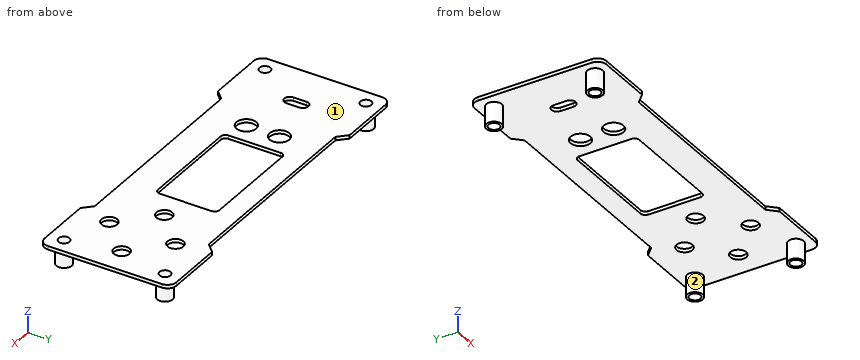
from build123d import *

# Parameters (mm, degrees)
PAD_DEPTH       = 0.8
POCKET_DEPTH    = 0.801
POCKET001_DEPTH = 0.801
SKETCH002_R     = 2.25
POCKET002_DEPTH = 0.801
SKETCH003_R     = 1.8
POCKET003_DEPTH = 0.801
SKETCH004_R     = 1.75
PAD001_DEPTH    = 4.5
SKETCH005_R     = 1.25
POCKET004_DEPTH = 5.301


with BuildPart() as part:
    # PCB_Sketch_76c7 → Pad (new body)
    with BuildSketch(Plane.XY):
        with BuildLine():
            Line((80, 28), (80, 2))
            ThreePointArc((80, 2), (79.414214, 0.585786), (78, 0))
            Line((78, 0), (65, 0))
            Line((65, 0), (63, 2))
            Line((63, 2), (17, 2))
            Line((17, 2), (15, 0))
            Line((15, 0), (2, 0))
            ThreePointArc((2, 0), (0.585786, 0.585786), (0, 2))
            Line((0, 2), (0, 28))
            ThreePointArc((0, 28), (0.585786, 29.414214), (2, 30))
            Line((2, 30), (15, 30))
            Line((17, 28), (15, 30))
            Line((63, 28), (17, 28))
            Line((63, 28), (65, 30))
            Line((65, 30), (78, 30))
            ThreePointArc((78, 30), (79.414214, 29.414214), (80, 28))
        make_face()
    extrude(amount=PAD_DEPTH)

    # Sketch (on Face18 of Pad) → Pocket (cut, through all)
    with BuildSketch(Plane.XY.offset(0.8)):
        with BuildLine():
            ThreePointArc((28.54066, 23.15), (27.79066, 22.83934), (27.48, 22.08934))
            Line((27.48, 10.21066), (27.48, 22.08934))
            ThreePointArc((27.48, 10.21066), (27.79066, 9.46066), (28.54066, 9.15))
            Line((51.41934, 9.15), (28.54066, 9.15))
            ThreePointArc((51.41934, 9.15), (52.16934, 9.46066), (52.48, 10.21066))
            Line((52.48, 22.08934), (52.48, 10.21066))
            ThreePointArc((52.48, 22.08934), (52.16934, 22.83934), (51.41934, 23.15))
            Line((28.54066, 23.15), (51.41934, 23.15))
        make_face()
    extrude(amount=-POCKET_DEPTH, mode=Mode.SUBTRACT)

    # Sketch001 (on Face5 of Pocket) → Pocket001 (cut, through all)
    with BuildSketch(Plane.XY.offset(0.8)):
        with BuildLine():
            ThreePointArc((11.65, 16.5), (10.4, 17.75), (9.15, 16.5))
            Line((9.15, 16.5), (9.15, 13.5))
            ThreePointArc((9.15, 13.5), (10.4, 12.25), (11.65, 13.5))
            Line((11.65, 13.5), (11.65, 16.5))
        make_face()
    extrude(amount=-POCKET001_DEPTH, mode=Mode.SUBTRACT)

    # Sketch002 (on Face5 of Pocket001) → Pocket002 (cut, through all)
    with BuildSketch(Plane.XY.offset(0.8)):
        with Locations((22.575, 18.77)):
            Circle(SKETCH002_R)
        with Locations((22.575, 11.22)):
            Circle(SKETCH002_R)
    extrude(amount=-POCKET002_DEPTH, mode=Mode.SUBTRACT)

    # Sketch003 (on Face5 of Pocket002) → Pocket003 (cut, through all)
    with BuildSketch(Plane.XY.offset(0.8)):
        with Locations((66.275, 22.47)):
            Circle(SKETCH003_R)
        with Locations((74.025, 15.07)):
            Circle(SKETCH003_R)
        with Locations((58.525, 15.07)):
            Circle(SKETCH003_R)
        with Locations((66.275, 7.42)):
            Circle(SKETCH003_R)
    extrude(amount=-POCKET003_DEPTH, mode=Mode.SUBTRACT)

    # Sketch004 (on Face4 of Pocket003) → Pad001 (join)
    with BuildSketch(Plane(origin=(0, 0, 0), x_dir=(1, 0, 0), z_dir=(0, 0, -1))):
        with Locations((3.5, -26.5)):
            Circle(SKETCH004_R)
        with Locations((3.5, -3.5)):
            Circle(SKETCH004_R)
        with Locations((76.5, -3.5)):
            Circle(SKETCH004_R)
        with Locations((76.5, -26.5)):
            Circle(SKETCH004_R)
    extrude(amount=PAD001_DEPTH)

    # Sketch005 (on Face5 of Pad001) → Pocket004 (cut, through all)
    with BuildSketch(Plane.XY.offset(0.8)):
        with Locations((3.5, 26.5)):
            Circle(SKETCH005_R)
        with Locations((3.5, 3.5)):
            Circle(SKETCH005_R)
        with Locations((76.5, 26.5)):
            Circle(SKETCH005_R)
        with Locations((76.5, 3.5)):
            Circle(SKETCH005_R)
    extrude(amount=-POCKET004_DEPTH, mode=Mode.SUBTRACT)


solid = part.part
Work out the finished part from the listing and answer in its coordinate system (mm). Face numbers are marked on the shaded views. Give positions to 0.01 mm unless a question says otherwise; leave off trailing zeros. Write each loop counter-clockwise with the first axis right and the second up, starting at its lowest first coordinate (ties: lowest second). Pieces come first, ordered by that corner, then holes. Notation, with made-up numbers: M -27.75,74.25 L 5.25,74.25 A23 cw 5.25,99.25 Z; hole C -31,74.5 d6. An arc over 180 degrees is marked long. Answer as CSV lines item,"result".
Q1. A cutting plane is placed at A-A on z = -1.45. Write down the section's boundary in (x, y).
A:
outline,"C 3.5,3.5 d3.5; C 3.5,26.5 d3.5; C 76.5,3.5 d3.5; C 76.5,26.5 d3.5; hole C 3.5,3.5 d2.5; hole C 3.5,26.5 d2.5; hole C 76.5,3.5 d2.5; hole C 76.5,26.5 d2.5"
Q2. The mould has two halves that part along Y. Classify the marked faces 1 and 2: +Y half, -Y half, draft (parallel to the pull), parting line (faces both ways), or undercut.
A:
face 1,"draft"
face 2,"undercut"
Q3. A cutting plane is placed at C-C on y = 7.42. Write down the section's boundary in (x, z) (3 decimals), plus the area to 3 significant figures.
A:
outline,"M 0,0 L 64.475,0 L 64.475,0.8 L 0,0.8 Z; M 68.075,0 L 80,0 L 80,0.8 L 68.075,0.8 Z"
area,"61.1 mm²"
Q4. A cutting plane is placed at B-B on x = 3.5. Write down the section's boundary in (y, z), plus the area to 3 significant figures.
A:
outline,"M 0,0 L 1.75,0 L 1.75,-4.5 L 2.25,-4.5 L 2.25,0.8 L 0,0.8 Z; M 4.75,-4.5 L 5.25,-4.5 L 5.25,0 L 24.75,0 L 24.75,-4.5 L 25.25,-4.5 L 25.25,0.8 L 4.75,0.8 Z; M 27.75,-4.5 L 28.25,-4.5 L 28.25,0 L 30,0 L 30,0.8 L 27.75,0.8 Z"
area,"29.0 mm²"
Q5. Find the intervals of material crossed by probe 1 along Y at (x, z) = (3.5, -1.8); probe 2 along Y at (x, z) = (38, 0.5); probe 3 along X at (y, z) = (27, -3.6), in increasing order. Write a range as [from, to].
A:
probe 1,"y = [1.75, 2.25], [4.75, 5.25], [24.75, 25.25], [27.75, 28.25]"
probe 2,"y = [2, 9.15], [23.15, 28]"
probe 3,"x = [1.82, 2.35], [4.65, 5.18], [74.82, 75.35], [77.65, 78.18]"
Q6. A cutting plane is placed at D-D on y = 11.22. Write down the section's boundary in (x, z) (3 decimals).
A:
outline,"M 0,0 L 20.325,0 L 20.325,0.8 L 0,0.8 Z; M 24.825,0 L 27.48,0 L 27.48,0.8 L 24.825,0.8 Z; M 52.48,0 L 80,0 L 80,0.8 L 52.48,0.8 Z"
Q7. Given P1, Ø3, axis at x = 47, z = 0, coming from the +Y side; P2, Ø3, axis at x = 58.525, y = 15.07, coming from the -Z side; P3, Ø4, axis at x = 59.5, y = 21, coming from the -Z side; P4, Ø0.6, axis at x = 30.5, z = 0.5, coming from the -Y side, each flat-ended and moving along its own axis, determine where each tip first touches the part or whether it passes through.
A:
P1,"stops at y = 28"
P2,"passes through"
P3,"stops at z = 0"
P4,"stops at y = 2"
